Work out the finished part from the listing and answer in its coordinate system (mm). A direction names the side the tool comes from. Coordinates: 2 decimals unless noted, no trailing zeros. Loops run counter-clockwise (first coordinate to the right, second up) from the corner with the lowest first, then second, coordinate; pieces in that order, holes last. Notation, with made-up numbers: (74, -30) -> (132, -30) arc R25 cw to (132, -2) -> close; hole circle Ø6 at (-8.75, 57.5). An arc over 180 degrees is marked (long way). One line per question, with ' | ' between items.
```python
from build123d import *

# Parameters (mm, degrees)
F1_DEPTH  = 125
F2_R      = 1.85
F3_DEPTH  = 4
F4_W      = 7
F4_H      = 1
F4_W_2    = 13.5
F4_W_3    = 10.669845
F5_DEPTH  = 3
F7_R      = 6
F8_DEPTH  = 25
F10_R     = 6
F11_DEPTH = 25


with BuildPart() as f1:
    # F0 (on Front) → F1 (new body)
    with BuildSketch(Plane.XZ):
        Polygon((27.424138, 47.5), (-27.424138, 47.5), (-23.960036, 41.5), (23.960036, 41.5), align=None)
    extrude(amount=F1_DEPTH)

    # F2 (on face) → F3 (cut)
    with BuildSketch(Plane(origin=(0, 0, 41.5), x_dir=(1, 0, 0), z_dir=(0, 0, -1))):
        with BuildLine():
            ThreePointArc((-13.830018, 120), (-11.980018, 118.15), (-10.130018, 120))
            Line((-10.130018, 120), (-13.830018, 120))
        make_face()
        with BuildLine():
            Line((-13.830018, 120), (-10.130018, 120))
            ThreePointArc((-10.130018, 120), (-11.980018, 121.85), (-13.830018, 120))
        make_face()
        with Locations((11.980018, 120)):
            Circle(F2_R)
        with BuildLine():
            ThreePointArc((-13.830018, 23), (-11.980018, 21.15), (-10.130018, 23))
            Line((-10.130018, 23), (-13.830018, 23))
        make_face()
        with BuildLine():
            Line((-13.830018, 23), (-10.130018, 23))
            ThreePointArc((-10.130018, 23), (-11.980018, 24.85), (-13.830018, 23))
        make_face()
        with Locations((11.980018, 23)):
            Circle(F2_R)
    extrude(amount=-F3_DEPTH, mode=Mode.SUBTRACT)

    # F4 (on face) → F5 (join)
    with BuildSketch(Plane.XY.offset(47.5)):
        with Locations((3.868914, -61.811117)):
            Rectangle(F4_W, F4_H)
        with BuildLine():
            ThreePointArc((1.113392, -63.582205), (-0.367617, -63.596068), (0.368914, -62.311117))
            Line((0.368914, -62.311117), (0.368914, -61.311117))
            ThreePointArc((0.368914, -61.311117), (-1.08188, -64.318326), (2.174842, -63.582205))
            Line((2.174842, -63.582205), (1.113392, -63.582205))
        make_face()
        with BuildLine():
            ThreePointArc((-4.330444, -62.004982), (-7.367157, -63.429113), (-6.131086, -60.311117))
            Line((-6.131086, -60.311117), (-6.131086, -59.311117))
            ThreePointArc((-6.131086, -59.311117), (-8.074487, -64.136422), (-3.329243, -62.004982))
            Line((-3.329243, -62.004982), (-4.330444, -62.004982))
        make_face()
        with Locations((0.618914, -59.811117)):
            Rectangle(F4_W_2, F4_H)
        with Locations((2.000717, -57.811117)):
            Rectangle(F4_W_3, F4_H)
        with BuildLine():
            ThreePointArc((-3.334205, -57.311117), (-4.397356, -55.372555), (-2.191203, -55.518156))
            Line((-2.191203, -55.518156), (-1.248077, -55.518156))
            ThreePointArc((-1.248077, -55.518156), (-5.077231, -54.833641), (-3.334205, -58.311117))
            Line((-3.334205, -58.311117), (-3.334205, -57.311117))
        make_face()
    extrude(amount=F5_DEPTH)

    # F7 (on face) → F8 (cut)
    with BuildSketch(Plane(origin=(-23.960036, 0, 41.5), x_dir=(0.866025, 0, 0.5), z_dir=(0.5, 0, -0.866025))):
        with Locations((0, 62.5)):
            Circle(F7_R)
    extrude(amount=F8_DEPTH, mode=Mode.SUBTRACT)

    # F10 (on face) → F11 (cut)
    with BuildSketch(Plane(origin=(23.960036, 0, 41.5), x_dir=(0.866025, 0, -0.5), z_dir=(0.5, 0, 0.866025))):
        with Locations((0, -62.5)):
            Circle(F10_R)
    extrude(amount=-F11_DEPTH, mode=Mode.SUBTRACT)


solid = f1.part
```
1) Find section B-B (y = -103.5). Write down the section's boundary in (x, z).
Check values:
outline: (-27.42, 47.5) -> (-23.96, 41.5) -> (23.96, 41.5) -> (27.42, 47.5) -> close
2) Find section A-A (y = -23). Write down the section's boundary in (x, z), plus the area to 3 significant figures.
Check values:
outline: (-27.42, 47.5) -> (-23.96, 41.5) -> (-13.83, 41.5) -> (-13.83, 45.5) -> (-10.13, 45.5) -> (-10.13, 41.5) -> (10.13, 41.5) -> (10.13, 45.5) -> (13.83, 45.5) -> (13.83, 41.5) -> (23.96, 41.5) -> (27.42, 47.5) -> close | area: 279 mm^2
3) Flat-ended cylindrical pins translate along their axes: pin 1 (3 mm diameter, centred on x = 5.5, y = -71, fed in from +Z); pin 2 (0.8 mm diameter, centred on y = -59.5, z = 48.5, fed in from +X); pin 3 (5 mm diameter, centred on x = 15.5, z = 49.5, fed in from +Y); pin 4 (2.5 mm diameter, centred on x = 3, z = 49, fed in from -Y). Find the tip coordinate at first contact, or state that the pin passes through.
Check values:
pin 1: stops at z = 47.5 | pin 2: stops at x = 7.37 | pin 3: stops at y = 0 | pin 4: stops at y = -64.4
4) Find the intervals of material crossed by line 1 along X through (y, z) = (-120, 44.3); line 2 along Y through (x, z) = (-5, 49.5); line 3 along X through (y, z) = (-23, 42.9), in increasing order.
Check values:
line 1: x = -25.58 to -13.83, -10.13 to 10.13, 13.83 to 25.58 | line 2: y = -64.68 to -63.52, -60.31 to -59.31, -57.53 to -54.74 | line 3: x = -24.77 to -13.83, -10.13 to 10.13, 13.83 to 24.77
5) For faces 1 (the face through (-1.12, -64.27, 48.98)), 2 (the face through (2, -62, 50.5)), 3 (the face through (4, -62.311, 49)), 4 (the face through (-12.221, -121.834, 43.472)), determine the directions among +Z, -Z, +X, -X, +Y, -Y from which every point of the face is accessible in a straight line to the end or side of a thin tool.
Check values:
face 1: +Z | face 2: +Z, +X, -X, +Y, -Y | face 3: +Z, +X | face 4: -Z
